Answer from the drawing. Dimensions are ordinates in mm from the lowest x, y and z of the part. Give positions to 0.01 mm unless a question says otherwise; leave off trailing zeros. Loops run counter-clockwise (first coordinate to the right, second up) from the corner with the lowest first, then second, coordinate; pieces in that order, holes last. Notation, with made-up numbers: M -10,23.5 L 47,23.5 A27 cw 47,39.5 Z; hole C 16.25,75 d10. An arc over 180 degrees is marked long. Use a Markdown table: item, result.
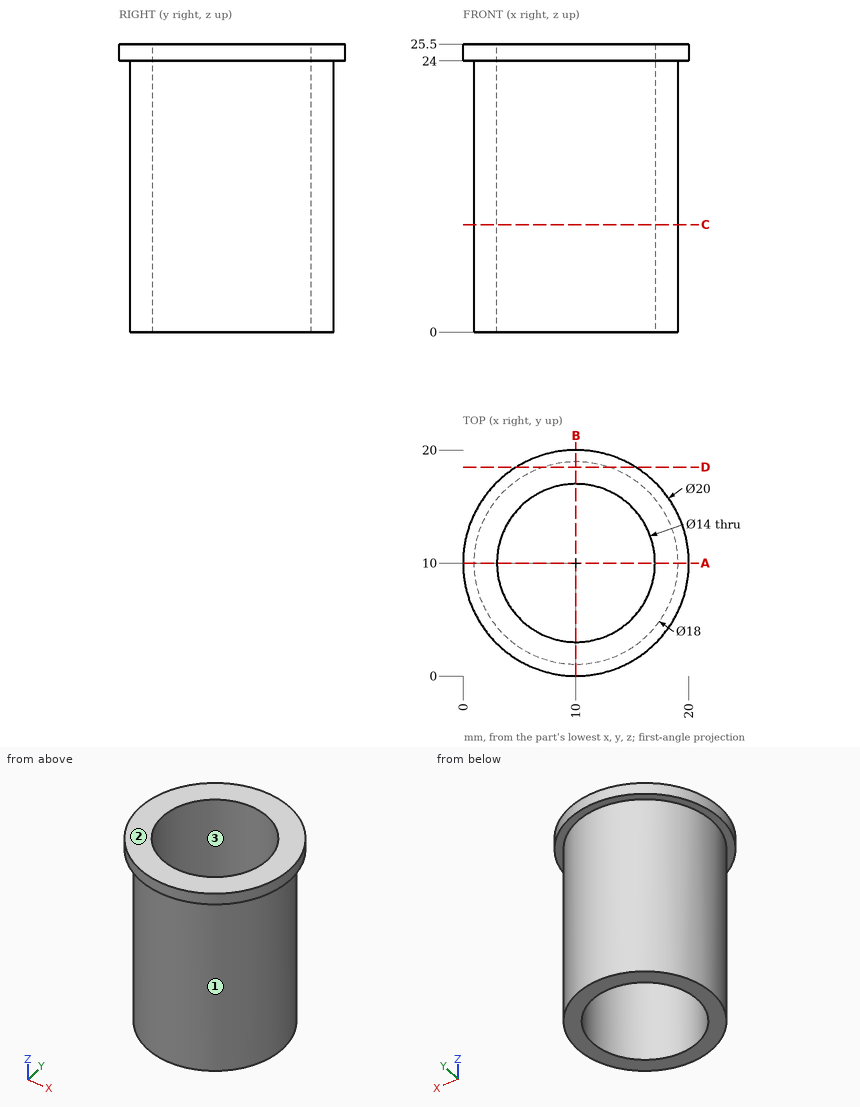
(1) Given P1, Ø2, axis at x = 2, z = 16.5, coming from the -Y side; P2, Ø8, axis at y = 7, z = 10.5, coming from the +X side; P3, Ø1.5, axis at x = 12.5, z = 12, coming from the -Y side, each flat-ended and moving along its own axis, determine where each tip first touches the part or whether it passes through.
Entries:
| item | result |
|---|---|
| P1 | stops at y = 4.34 |
| P2 | stops at x = 19 |
| P3 | stops at y = 1.17 |
(2) A cutting plane is placed at A-A (y = 10). Write down the section's boundary in (x, z).
Entries:
| item | result |
|---|---|
| outline | M 0,24 L 1,24 L 1,0 L 3,0 L 3,25.5 L 0,25.5 Z; M 17,0 L 19,0 L 19,24 L 20,24 L 20,25.5 L 17,25.5 Z |
(3) A cutting plane is placed at D-D (y = 18.5). Write down the section's boundary in (x, z).
Entries:
| item | result |
|---|---|
| outline | M 4.73,24 L 7.04,24 L 7.04,0 L 12.96,0 L 12.96,24 L 15.27,24 L 15.27,25.5 L 4.73,25.5 Z |
(4) Consider probe 1 along Y at (x, z) = (10, 15.5); probe 2 along X at (y, z) = (8.5, 19.25); probe 3 along Y at (x, z) = (5, 17). Determine where each line is inside the solid, lowest interval first. Write a range as [from, to].
Entries:
| item | result |
|---|---|
| probe 1 | y = [1, 3], [17, 19] |
| probe 2 | x = [1.13, 3.16], [16.84, 18.87] |
| probe 3 | y = [2.52, 5.1], [14.9, 17.48] |
(5) The mould has two halves that part along X. Classify the marked faces 1, 2 and 3: released by +X, released by -X, zero draft, split by the parting line, or undercut.
Entries:
| item | result |
|---|---|
| face 1 | split by the parting line |
| face 2 | zero draft |
| face 3 | undercut |
(6) A cutting plane is placed at C-C (z = 9.5). Write down the section's boundary in (x, y).
Entries:
| item | result |
|---|---|
| outline | C 10,10 d18; hole C 10,10 d14 |
